Work out the finished part from the listing and answer in its coordinate system (mm). Round coordinates to 2 decimals unless told otherwise and drop trailing zeros. Order: outer loops, then holes, each group sorted by start corner. A loop starts at its lowest first (then second) coordinate and runs counter-clockwise, first axis right, second up. Notation, with made-up numbers: M 54.5,-23 L 81.5,-23 A26 cw 81.5,15 Z; hole C -12,35 d10. An arc over 180 degrees is marked long. Answer as a JSON object with one key per item and string values. Group by question number.
from build123d import *

# Parameters (mm, degrees)
SKETCH_1_R               = 5.5
EXTRUDE_1_DEPTH          = 1.5
CUT_EXTRUDE_1_DEPTH      = 166.102998156
CUT_EXTRUDE_1_DEPTH_BACK = 10
SKETCH_2_R               = 1.6
SKETCH_2_R_2             = 7.5


with BuildPart() as part:
    # 草图1 → 凸台-拉伸1 (new, symmetric)
    with BuildSketch(Plane.XY):
        with BuildLine():
            Line((-10, 25), (-120, 25))
            ThreePointArc((-120, 25), (-130.606601718, 20.606601718), (-135, 10))
            Line((-135, 10), (-135, -35))
            Line((-135, -35), (-135, -80))
            ThreePointArc((-135, -80), (-130.606601718, -90.606601718), (-120, -95))
            Line((-120, -95), (-110, -95))
            Line((-110, -95), (-100, -95))
            ThreePointArc((-100, -95), (-89.393398282, -90.606601718), (-85, -80))
            Line((-85, -80), (-85, -40))
            ThreePointArc((-85, -40), (-80.606601718, -29.393398282), (-70, -25))
            Line((-70, -25), (-60, -25))
            Line((-60, -25), (-60, -30))
            Line((-60, -30), (-45, -30))
            Line((-45, -30), (-20, -30))
            Line((-20, -30), (-20, -25))
            Line((-20, -25), (0, -25))
            Line((0, -25), (20, -25))
            Line((20, -25), (20, -30))
            Line((20, -30), (45, -30))
            Line((45, -30), (60, -30))
            Line((60, -30), (60, -25))
            Line((60, -25), (70, -25))
            ThreePointArc((70, -25), (80.606601718, -29.393398282), (85, -40))
            Line((85, -40), (85, -80))
            ThreePointArc((85, -80), (89.393398282, -90.606601718), (100, -95))
            Line((100, -95), (120, -95))
            ThreePointArc((120, -95), (130.606601718, -90.606601718), (135, -80))
            Line((135, -80), (135, -35))
            Line((135, -35), (135, 10))
            ThreePointArc((135, 10), (130.606601718, 20.606601718), (120, 25))
            Line((120, 25), (10, 25))
            Line((10, 25), (10, 30))
            Line((10, 30), (-10, 30))
            Line((-10, 30), (-10, 25))
        make_face()
        with Locations((-120, -86.5)):
            Circle(SKETCH_1_R, mode=Mode.SUBTRACT)
        with BuildLine():
            ThreePointArc((-94.5, -86.5), (-100, -92), (-105.5, -86.5))
            ThreePointArc((-105.5, -86.5), (-100, -81), (-94.5, -86.5))
        make_face(mode=Mode.SUBTRACT)
        with Locations((100, -86.5)):
            Circle(SKETCH_1_R, mode=Mode.SUBTRACT)
        with Locations((120, -86.5)):
            Circle(SKETCH_1_R, mode=Mode.SUBTRACT)
    extrude(amount=EXTRUDE_1_DEPTH, both=True)

    # 草图2 → 切除-拉伸1 (cut, two sides: drawn at the far end of the back side and taken through both)
    with BuildSketch(Plane.XY.offset(1.5).offset(-CUT_EXTRUDE_1_DEPTH_BACK)):
        with BuildLine():
            Line((80, 15), (-80, 15))
            ThreePointArc((-80, 15), (-95, 0), (-80, -15))
            Line((-80, -15), (80, -15))
            ThreePointArc((80, -15), (95, 0), (80, 15))
        make_face()
        with Locations(Location((-110, -76, 0), (0, 0, 180))):
            Circle(SKETCH_2_R)
        with BuildLine():
            ThreePointArc((-120, -61), (-117.071067812, -68.071067812), (-110, -71))
            ThreePointArc((-110, -71), (-102.928932188, -68.071067812), (-100, -61))
            Line((-100, -61), (-100, -21))
            ThreePointArc((-100, -21), (-110, -11), (-120, -21))
            Line((-120, -21), (-120, -61))
        make_face()
        with Locations(Location((-90, -20, 0), (0, 0, 180))):
            Circle(SKETCH_2_R)
        with BuildLine():
            ThreePointArc((120, -21), (110, -11), (100, -21))
            Line((100, -21), (100, -61))
            ThreePointArc((100, -61), (110, -71), (120, -61))
            Line((120, -61), (120, -21))
        make_face()
        with Locations(Location((-107.5, -2.5, 0), (0, 0, 180))):
            Circle(SKETCH_2_R)
        with Locations(Location((90, -20, 0), (0, 0, 180))):
            Circle(SKETCH_2_R)
        with Locations(Location((107.5, -2.5, 0), (0, 0, 180))):
            Circle(SKETCH_2_R)
        with Locations(Location((-125, 15, 0), (0, 0, 180))):
            Circle(SKETCH_2_R)
        with Locations(Location((-120, 0, 0), (0, 0, 180))):
            Circle(SKETCH_2_R_2)
        with Locations(Location((125, 15, 0), (0, 0, 180))):
            Circle(SKETCH_2_R)
        with Locations(Location((120, 0, 0), (0, 0, 180))):
            Circle(SKETCH_2_R_2)
        with Locations(Location((110, -76, 0), (0, 0, 180))):
            Circle(SKETCH_2_R)
    extrude(amount=CUT_EXTRUDE_1_DEPTH + CUT_EXTRUDE_1_DEPTH_BACK, mode=Mode.SUBTRACT)


solid = part.part
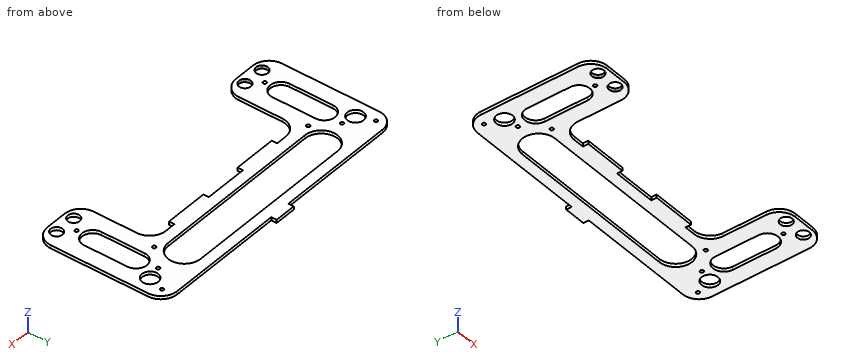
Item 1: Find section A-A (x = -17). Give the vertices of the cut face in (y, z).
Item 2: Each of these flat-tipped pins is pushed along its axis until it touches: pin 1 (24 mm diameter, centred on x = -120, y = 0, fed in from -Z); pin 2 (1.5 mm diameter, centred on x = -16.5, z = -0.5, fed in from +Y); pin 3 (10 mm diameter, centred on x = -100, y = -86.5, fed in from -Z); pin 4 (1.5 mm diameter, centred on y = 26.5, z = -0.5, fed in from +X). Where does it stop, or does it pass through?
Item 3: Consider L1, parallel to X at y = -76, z = -0.55; L2, parallel to X at y = -53, z = -0.5; L3, parallel to X at y = -22, z = -0.75. Determine where each line is inside the solid, lowest interval first.
Item 4: Find section B-B (z = 0.95). Give the number of separate pieces and of enclosed holes in the cut face, and give its area (3 significant figures).
Responses:
{
 "1": {"outline": "M -25,-1.5 L -15,-1.5 L -15,1.5 L -25,1.5 Z; M 15,-1.5 L 25,-1.5 L 25,1.5 L 15,1.5 Z"},
 "2": {"pin 1": "stops at z = -1.5", "pin 2": "stops at y = 25", "pin 3": "passes through", "pin 4": "stops at x = 10"},
 "3": {"L1": "x = -135 to -111.6, -108.4 to -85, 85 to 108.4, 111.6 to 135", "L2": "x = -135 to -120, -100 to -85, 85 to 100, 120 to 135", "L3": "x = -135 to -120, -100 to 100, 120 to 135"},
 "4": {"separate pieces": "1", "enclosed holes": "17", "area": "12,300 mm^2"}
}
